CAD build for the part. Positions are in the model's coordinates, mm. A direction names the side the tool comes from. Round coordinates to 2 decimals unless told otherwise and drop trailing zeros. Write each loop counter-clockwise with the first axis right and the second up, starting at its lowest first coordinate (ties: lowest second). Pieces come first, ordered by that corner, then holes. Notation, with made-up numbers: (7, 14.5) - (51, 14.5) arc R21 cw to (51, 39.5) - close; hole circle Ø4 at (67, 26.25). An arc over 180 degrees is marked (long way). Answer in a Markdown table with one row per item.
```python
from build123d import *

# Parameters (mm, degrees)
F0_W     = 176.2125
F0_H     = 100.076
F1_DEPTH = 64.77
F2_W     = 173.6725
F2_H     = 97.536
F3_DEPTH = 1.27
F5_DEPTH = 39.37


with BuildPart() as f1:
    # F0 (on Top) → F1 (new body, symmetric)
    with BuildSketch(Plane.XY):
        Rectangle(F0_W, F0_H)
    extrude(amount=F1_DEPTH, both=True)

    # F2 (on face) → F3 (join)
    with BuildSketch(Plane.XY.offset(64.77)):
        Rectangle(F2_W, F2_H)
    extrude(amount=F3_DEPTH)

    # F4 (on face) → F5 (join)
    with BuildSketch(Plane.XY.offset(66.04)):
        Polygon((61.43625, 48.768), (-61.43625, 48.768), (-61.43625, 23.368), (-86.83625, 23.368), (-86.83625, -48.768), (86.83625, -48.768), (86.83625, 23.368), (61.43625, 23.368), align=None)
    extrude(amount=F5_DEPTH)


solid = f1.part
```
Q1. Saw through at A-A on y = 38.5. List the corners of the cut face in (x, z), then the cut area to 3 significant figures.
Computed:
| item | result |
|---|---|
| outline | (-88.11, -64.77) - (88.11, -64.77) - (88.11, 64.77) - (86.84, 64.77) - (86.84, 66.04) - (61.44, 66.04) - (61.44, 105.41) - (-61.44, 105.41) - (-61.44, 66.04) - (-86.84, 66.04) - (-86.84, 64.77) - (-88.11, 64.77) - close |
| area | 27,900 mm2 |
Q2. Drill centre lines: line 1 (X direction, y = 34, z = 91); line 2 (X direction, y = -5, z = 89.5); line 3 (Z direction, x = 69, y = 43.5). Where is each one in solid material? Low to high.
Computed:
| item | result |
|---|---|
| line 1 | x = -61.44 to 61.44 |
| line 2 | x = -86.84 to 86.84 |
| line 3 | z = -64.77 to 66.04 |
Q3. 3-axis set-ups, long thin cutter, end or side, ignore diameter. For faces 1 (the flat face through (-1, -48.768, 85)), 2 (the flat face through (1, 48.768, 85)), 3 (the flat face through (61.436, 36, 85)): which of +Z, -Z, +X, -X, +Y, -Y reach the whole face in a straight line?
Computed:
| item | result |
|---|---|
| face 1 | +Z, +X, -X, -Y |
| face 2 | +Z, +X, -X, +Y |
| face 3 | +Z, +X, +Y |
Q4. Saw through at C-C on x = 70. List the corners of the cut face in (y, z).
Computed:
| item | result |
|---|---|
| outline | (-50.04, -64.77) - (50.04, -64.77) - (50.04, 64.77) - (48.77, 64.77) - (48.77, 66.04) - (23.37, 66.04) - (23.37, 105.41) - (-48.77, 105.41) - (-48.77, 64.77) - (-50.04, 64.77) - close |
Q5. Saw through at B-B on z = 90.5. List the corners of the cut face in (x, y).
Computed:
| item | result |
|---|---|
| outline | (-86.84, -48.77) - (86.84, -48.77) - (86.84, 23.37) - (61.44, 23.37) - (61.44, 48.77) - (-61.44, 48.77) - (-61.44, 23.37) - (-86.84, 23.37) - close |
Q6. Flat gauge pins, fed straight in: pin 1 (20.5 mm diameter, centred on y = -8, z = 83.5, fed in from -X); pin 2 (7.5 mm diameter, centred on x = 73, y = 35.5, fed in from +Z); pin 3 (20.5 mm diameter, centred on y = 2.5, z = 78, fed in from +X). Where does each tip first touch, or does it go through?
Computed:
| item | result |
|---|---|
| pin 1 | stops at x = -86.84 |
| pin 2 | stops at z = 66.04 |
| pin 3 | stops at x = 86.84 |
